```python
from build123d import *

# Parameters (mm, degrees)
ESQUISSE1_R        = 150
ESQUISSE1_R_2      = 1.5
ESQUISSE1_W        = 5
ESQUISSE1_H        = 5
BOSS_EXTRU_1_DEPTH = 5
CONG_1_R           = 1.5


with BuildPart() as part:
    # Esquisse1 → Boss.-Extru.1 (new body)
    with BuildSketch(Plane.XY):
        Circle(ESQUISSE1_R)
        with Locations((-135, 0)):
            Circle(ESQUISSE1_R_2, mode=Mode.SUBTRACT)
        with Locations((0, 135)):
            Circle(ESQUISSE1_R_2, mode=Mode.SUBTRACT)
        with Locations((135, 0)):
            Circle(ESQUISSE1_R_2, mode=Mode.SUBTRACT)
        with Locations((0, -135)):
            Circle(ESQUISSE1_R_2, mode=Mode.SUBTRACT)
        with BuildLine():
            Line((-20, 118.321595662), (-20, 20))
            Line((-20, 20), (-21.893135369, 20))
            Line((-21.893135369, 20), (-26.893135369, -10))
            Line((-26.893135369, -10), (-31.893135369, 20))
            Line((-31.893135369, 20), (-55.504004396, 20))
            Line((-55.504004396, 20), (-60.504004396, -10))
            Line((-60.504004396, -10), (-65.504004396, 20))
            Line((-65.504004396, 20), (-89.114873423, 20))
            Line((-89.114873423, 20), (-94.114873423, -10))
            Line((-94.114873423, -10), (-99.114873423, 20))
            Line((-99.114873423, 20), (-118.321595662, 20))
            ThreePointArc((-118.321595662, 20), (-84.852813742, 84.852813742), (-20, 118.321595662))
        make_face(mode=Mode.SUBTRACT)
        with BuildLine():
            Line((20, 118.321595662), (20, 20))
            Line((20, 20), (21.893135369, 20))
            Line((21.893135369, 20), (26.893135369, -10))
            Line((26.893135369, -10), (31.893135369, 20))
            Line((31.893135369, 20), (55.504004396, 20))
            Line((55.504004396, 20), (60.504004396, -10))
            Line((60.504004396, -10), (65.504004396, 20))
            Line((65.504004396, 20), (89.114873423, 20))
            Line((89.114873423, 20), (94.114873423, -10))
            Line((94.114873423, -10), (99.114873423, 20))
            Line((99.114873423, 20), (118.321595662, 20))
            ThreePointArc((118.321595662, 20), (84.852813742, 84.852813742), (20, 118.321595662))
        make_face(mode=Mode.SUBTRACT)
        with BuildLine():
            Line((118.321595662, -20), (20, -20))
            Line((20, -20), (20, -118.321595662))
            ThreePointArc((20, -118.321595662), (84.852813742, -84.852813742), (118.321595662, -20))
        make_face(mode=Mode.SUBTRACT)
        with BuildLine():
            Line((-20, -118.321595662), (-20, -20))
            Line((-20, -20), (-118.321595662, -20))
            ThreePointArc((-118.321595662, -20), (-84.852813742, -84.852813742), (-20, -118.321595662))
        make_face(mode=Mode.SUBTRACT)
        with Locations((-135, -7.5)):
            Rectangle(ESQUISSE1_W, ESQUISSE1_H, mode=Mode.SUBTRACT)
        with Locations((-135, 7.5)):
            Rectangle(ESQUISSE1_W, ESQUISSE1_H, mode=Mode.SUBTRACT)
        with Locations((-7.5, 135)):
            Rectangle(ESQUISSE1_W, ESQUISSE1_H, mode=Mode.SUBTRACT)
        with Locations((7.5, 135)):
            Rectangle(ESQUISSE1_W, ESQUISSE1_H, mode=Mode.SUBTRACT)
        with Locations((135, 7.5)):
            Rectangle(ESQUISSE1_W, ESQUISSE1_H, mode=Mode.SUBTRACT)
        with Locations((135, -7.5)):
            Rectangle(ESQUISSE1_W, ESQUISSE1_H, mode=Mode.SUBTRACT)
        with Locations((7.5, -135)):
            Rectangle(ESQUISSE1_W, ESQUISSE1_H, mode=Mode.SUBTRACT)
        with Locations((-7.5, -135)):
            Rectangle(ESQUISSE1_W, ESQUISSE1_H, mode=Mode.SUBTRACT)
    extrude(amount=BOSS_EXTRU_1_DEPTH)

    # Congé1
    cong_1_edges = [part.edges().sort_by_distance(p)[0] for p in [
        (-20, -20, 2.5),
        (-118.321595662, -20, 2.5),
        (-20, -118.321595662, 2.5),
        (20, -20, 2.5),
        (20, -118.321595662, 2.5),
        (118.321595662, -20, 2.5),
        (21.893135369, 20, 2.5),
        (26.893135369, -10, 2.5),
        (31.893135369, 20, 2.5),
        (55.504004396, 20, 2.5),
        (60.504004396, -10, 2.5),
        (65.504004396, 20, 2.5),
        (89.114873423, 20, 2.5),
        (94.114873423, -10, 2.5),
        (99.114873423, 20, 2.5),
        (118.321595662, 20, 2.5),
        (20, 118.321595662, 2.5),
        (-99.114873423, 20, 2.5),
        (-94.114873423, -10, 2.5),
        (-89.114873423, 20, 2.5),
        (-65.504004396, 20, 2.5),
        (-60.504004396, -10, 2.5),
        (-55.504004396, 20, 2.5),
        (-31.893135369, 20, 2.5),
        (-26.893135369, -10, 2.5),
        (-21.893135369, 20, 2.5),
        (-20, 118.321595662, 2.5),
        (-118.321595662, 20, 2.5),
    ]]
    fillet(cong_1_edges, radius=CONG_1_R)


solid = part.part
```
Geometry: final body of the model. Coordinates: model frame, mm. A direction names the side the tool comes from. Give positions to 0.01 mm unless a question says otherwise; leave off trailing zeros. Order: outer loops, then holes, each group sorted by start corner. A loop starts at its lowest first (then second) coordinate and runs counter-clockwise, first axis right, second up. Notation, with made-up numbers: (42, 35) -> (54, 35) arc R22 cw to (54, 54) -> close; hole circle Ø3 at (70.25, -21). An arc over 180 degrees is marked (long way). Write each question's results on one line, items separated by ' | '. Start each with the question number.
1) Section C-C (z = 2.15). Count the separate pieces of the cut face and the enclosed holes in it, then the cut area to 3 significant figures.
2) Section B-B (x = 78). Return loops of the section in (y, z).
3) Section A-A (y = 55). Return loops of the section in (x, z).
4) Set-up query: faces 4 (the flat face through (-2, 2, 5)), 5 (the cylindrical face through (84.1, -85.6, 2.5)). Return all of +Z, -Z, +X, -X, +Y, -Y with unobstructed straight access to the full face (end or side cutting, diameter ignored); none if empty.
5) First-contact query: pin 1 (1.5 mm diameter, centred on y = -135.5, z = 3.5, fed in from +X); pin 2 (2 mm diameter, centred on x = 42, z = 3, fed in from -Y); pin 3 (2 mm diameter, centred on x = -114, z = 3, fed in from -Y); pin 4 (3.5 mm diameter, centred on x = -135, y = 0, fed in from +Z). Flat tips, straight axial feed; report the tip coordinate or a pass-through.
6) Draft query along Y for faces 1 (the flat face through (-2, 2, 0)), 2 (the cylindrical face through (-85.6, -84.1, 2.5)), 3 (the cylindrical face through (-19.527, 148.724, 2.465)). Return one class per face: pulls with the +Y half, pulls with the -Y half, needs draft (parallel to the pull), parting line crosses it, or undercut.
7) Line query: line 1 (X direction, y = -135, z = 1.7); line 2 (Y direction, x = 0, z = 1.2). Output: solid intervals per line, ascending. Write a range as from..to.
Calculated:
1) separate pieces: 1 | enclosed holes: 16 | area: 41,900 mm2
2) outline: (-128.12, 0) -> (-91.19, 0) -> (-91.19, 5) -> (-128.12, 5) -> close; (-20, 0) -> (20, 0) -> (20, 5) -> (-20, 5) -> close; (91.19, 0) -> (128.12, 0) -> (128.12, 5) -> (91.19, 5) -> close
3) outline: (-139.55, 0) -> (-106.65, 0) -> (-106.65, 5) -> (-139.55, 5) -> close; (-20, 0) -> (20, 0) -> (20, 5) -> (-20, 5) -> close; (106.65, 0) -> (139.55, 0) -> (139.55, 5) -> (106.65, 5) -> close
4) face 4: +Z, +X, -X, +Y, -Y | face 5: +Z, -Z
5) pin 1: x = 65.9 | pin 2: y = -144.29 | pin 3: y = -98.65 | pin 4: z = 5
6) face 1: needs draft | face 2: undercut | face 3: parting line crosses it
7) line 1: -65.38..-10, -5..-1.5, 1.5..5, 10..65.38 | line 2: -150..-136.5, -133.5..133.5, 136.5..150
